```python
from build123d import *

# Parameters (mm, degrees)
SKETCH1_R           = 47
SKETCH1_R_2         = 2.25
BOSS_EXTRUDE1_DEPTH = 10
CUT_EXTRUDE1_DEPTH  = 3.86
SKETCH3_R           = 1.75
CUT_EXTRUDE2_DEPTH  = 67.751026958


with BuildPart() as part:
    # Sketch1 → Boss-Extrude1 (new body)
    with BuildSketch(Plane(origin=(0, 0, 0), x_dir=(0, 1, 0), z_dir=(0, 0, 1))):
        with Locations(Location((0, 0, 0), (0, 0, 270))):
            Circle(SKETCH1_R)
        with Locations(Location((0, 34.897005385, 0), (0, 0, 270))):
            Circle(SKETCH1_R_2, mode=Mode.SUBTRACT)
        with Locations(Location((0, -34.897005385, 0), (0, 0, 90))):
            Circle(SKETCH1_R_2, mode=Mode.SUBTRACT)
    extrude(amount=BOSS_EXTRUDE1_DEPTH)

    # Sketch2 → Cut-Extrude1 (cut)
    with BuildSketch(Plane.XY.offset(10)):
        with BuildLine():
            Line((24.33053856, 3.5), (12, 3.5))
            ThreePointArc((12, 3.5), (8.440790603, 3.996719292), (5.153570125, 5.448918697))
            ThreePointArc((5.153570125, 5.448918697), (-7.5, 0), (5.153570125, -5.448918697))
            ThreePointArc((5.153570125, -5.448918697), (8.440790603, -3.996719292), (12, -3.5))
            Line((12, -3.5), (24.33053856, -3.5))
            ThreePointArc((24.33053856, -3.5), (27.83053856, 0), (24.33053856, 3.5))
        make_face()
    extrude(amount=-CUT_EXTRUDE1_DEPTH, mode=Mode.SUBTRACT)

    # Sketch3 → Cut-Extrude2 (cut, through all)
    with BuildSketch(Plane.XY.offset(6.14)):
        Circle(SKETCH3_R)
        with Locations((20, 0)):
            Circle(SKETCH3_R)
        with Locations((24, 0)):
            Circle(SKETCH3_R)
    extrude(amount=-CUT_EXTRUDE2_DEPTH, mode=Mode.SUBTRACT)


solid = part.part
```
Can you work these out from the model? Positions are in its coordinate system, mm. A direction names the side the tool comes from. Round coordinates to 2 decimals unless told otherwise and drop trailing zeros. Loops run counter-clockwise (first coordinate to the right, second up) from the corner with the lowest first, then second, coordinate; pieces in that order, holes last. Notation, with made-up numbers: M 33.5,22 L 55.5,22 A10 cw 55.5,38 Z; hole C 64.25,-4.75 d10. An arc over 180 degrees is marked long. Write item = value, one per line. Start each with the question number.
(1) Suppose I cut it at B-B on z = 8.25. Write out the boundary of the cut face in (x, y).
(2) If we mould it in two halves opening along X, with no side actions, what happens to faces 1 (the face through (22.25, 0.08, 3.11)), 2 (the face through (-34.641, 31.765, 4.93)), 3 (the face through (6, 0, 6.14)), 4 (the face through (-1, -10, 10))? For each: released by +X, released by -X, zero draft, split by the parting line, or undercut.
(3) I need wall thicknesses on line 1 along Y through (x, z) = (0, 2.5); line 2 along Z through (x, y) = (12, 2.5); line 3 along Y through (x, z) = (25.5, 4.25). Which ranges of each line are inside material? Lowest first, please.
(4) Suppose I cut it at D-D on x = 20. Write out the boundary of the cut face in (y, z), plus the area to 3 significant figures.
(5) Suppose I cut it at C-C on x = 0. Write out the boundary of the cut face in (y, z).
(6) Which directions (+Z, -Z, +X, -X, +Y, -Y) give clear straight access to the entire face, cutting with the end or side of a thin tool? Please do faces 5 (the face through (-1, -10, 0)), 6 (the face through (8.489, 3.983, 8.097)).
(7) Suppose I cut it at A-A on y = 0. Write out the boundary of the cut face in (x, z), plus the area to 3 significant figures.
(8) I'm going to push flat-ended pins straight in: P1, Ø1, axis at y = 2.5, z = 5.5, coming from the +X side; P2, Ø4, axis at x = 20, y = 0, coming from the +Z side; P3, Ø4, axis at x = 34.9, y = 0, coming from the +Z side; P4, Ø4, axis at x = -16, z = 4, coming from the -Y side. Where does each tip first touch, or does it pass through?
Answer block:
q1.outline = C 0,0 d94; hole C -34.9,0 d4.5; hole M 5.15,-5.45 A13 cw 12,-3.5 L 24.33,-3.5 A3.5 ccw 24.33,3.5 L 12,3.5 A13 cw 5.15,5.45 A7.5 ccw long Z; hole C 34.9,0 d4.5
q2.face_1 = undercut
q2.face_2 = split by the parting line
q2.face_3 = undercut
q2.face_4 = zero draft
q3.line_1 = -47 to -1.75, 1.75 to 47
q3.line_2 = 0 to 6.14
q3.line_3 = -39.48 to -0.9, 0.9 to 39.48
q4.outline = M -42.53,0 L -1.75,0 L -1.75,6.14 L -3.5,6.14 L -3.5,10 L -42.53,10 Z; M 1.75,0 L 42.53,0 L 42.53,10 L 3.5,10 L 3.5,6.14 L 1.75,6.14 Z
q4.area = 802 mm²
q5.outline = M -47,0 L -1.75,0 L -1.75,6.14 L -7.5,6.14 L -7.5,10 L -47,10 Z; M 1.75,0 L 47,0 L 47,10 L 7.5,10 L 7.5,6.14 L 1.75,6.14 Z
q6.face_5 = -Z, +X, -X, +Y, -Y
q6.face_6 = +Z
q7.outline = M -47,0 L -37.15,0 L -37.15,10 L -47,10 Z; M -32.65,0 L -1.75,0 L -1.75,6.14 L -7.5,6.14 L -7.5,10 L -32.65,10 Z; M 1.75,0 L 18.25,0 L 18.25,6.14 L 1.75,6.14 Z; M 21.75,0 L 22.25,0 L 22.25,6.14 L 21.75,6.14 Z; M 25.75,0 L 32.65,0 L 32.65,10 L 27.83,10 L 27.83,6.14 L 25.75,6.14 Z; M 37.15,0 L 47,0 L 47,10 L 37.15,10 Z
q7.area = 649 mm²
q8.P1 = 46.96
q8.P2 = 6.14
q8.P3 = through
q8.P4 = -44.87
